from build123d import *

# Parameters (mm, degrees)
BASE_FLANGE1_DEPTH = 211
SKETCH10_R         = 1.75
EXTRUDE2_DEPTH     = 10


# Sheet-metal steps are written as plain solids
with BuildPart() as part:
    # Sketch1 → Base-Flange1 (new, symmetric)
    with BuildSketch(Plane.XY):
        with BuildLine():
            Line((0, 0), (21.9, 0))
            ThreePointArc((21.9, 0), (23.9, -2), (21.9, -4))
            Line((21.9, -4), (16.9, -4))
            Line((16.9, -4), (16.9, -3.5))
            Line((16.9, -3.5), (21.9, -3.5))
            ThreePointArc((21.9, -3.5), (23.4, -2), (21.9, -0.5))
            Line((21.9, -0.5), (0, -0.5))
            Line((0, -0.5), (0, 0))
        make_face()
    extrude(amount=BASE_FLANGE1_DEPTH, both=True)

    # Sketch10 → Extrude2 (cut)
    with BuildSketch(Plane(origin=(0, 0, 0), x_dir=(1, 0, 0), z_dir=(0, 1, 0))):
        with Locations(Location((5, 0, 0), (0, 0, 270))):
            Circle(SKETCH10_R)
        with Locations(Location((5, 196, 0), (0, 0, 270))):
            Circle(SKETCH10_R)
        with Locations(Location((5, -196, 0), (0, 0, 270))):
            Circle(SKETCH10_R)
    extrude(amount=-EXTRUDE2_DEPTH, mode=Mode.SUBTRACT)


solid = part.part
For this review, take the finished solid that the model builds, in its own axes (mm). A direction names the side the tool comes from. Give positions to 0.01 mm unless a question says otherwise; leave off trailing zeros. Loops run counter-clockwise (first coordinate to the right, second up) from the corner with the lowest first, then second, coordinate; pieces in that order, holes last.
Item 1: For line 1 along Y through (x, z) = (20, 41.5); line 2 along Y through (x, z) = (1.5, 103); line 3 along X through (y, z) = (-0.25, -196), list the stretches that pass through material, from the lowest coordinate up.
Item 2: Take a section at B-B, the plane y = -2. State the section outline as (x, z) points, and give its area (3 significant figures).
Item 3: Tool access review of faces 1 (the flat face through (11, -0.5, 3)), 2 (the flat face through (11, 0, 3)): name each direction out of +Z, -Z, +X, -X, +Y, -Y from which nothing blocks a thin tool from reaching the whole face with its end or side.
Item 4: Take a section at C-C, the plane x = 12.75. State the section outline as (y, z) points.
Item 5: Take a section at A-A, the plane z = -54. State the section outline as (x, y) points, and give its area (3 significant figures).
Calculated:
1. line 1: y = -4 to -3.5, -0.5 to 0
1. line 2: y = -0.5 to 0
1. line 3: x = 0 to 3.25, 6.75 to 22.87
2. outline: (23.4, -211) - (23.9, -211) - (23.9, 211) - (23.4, 211) - close
2. area: 211 mm2
3. face 1: +Z, -Z, -X
3. face 2: +Z, -Z, +X, -X, +Y
4. outline: (-0.5, -211) - (0, -211) - (0, 211) - (-0.5, 211) - close
5. outline: (0, -0.5) - (21.9, -0.5) arc R1.5 cw to (21.9, -3.5) - (16.9, -3.5) - (16.9, -4) - (21.9, -4) arc R2 ccw to (21.9, 0) - (0, 0) - close
5. area: 16.2 mm2
